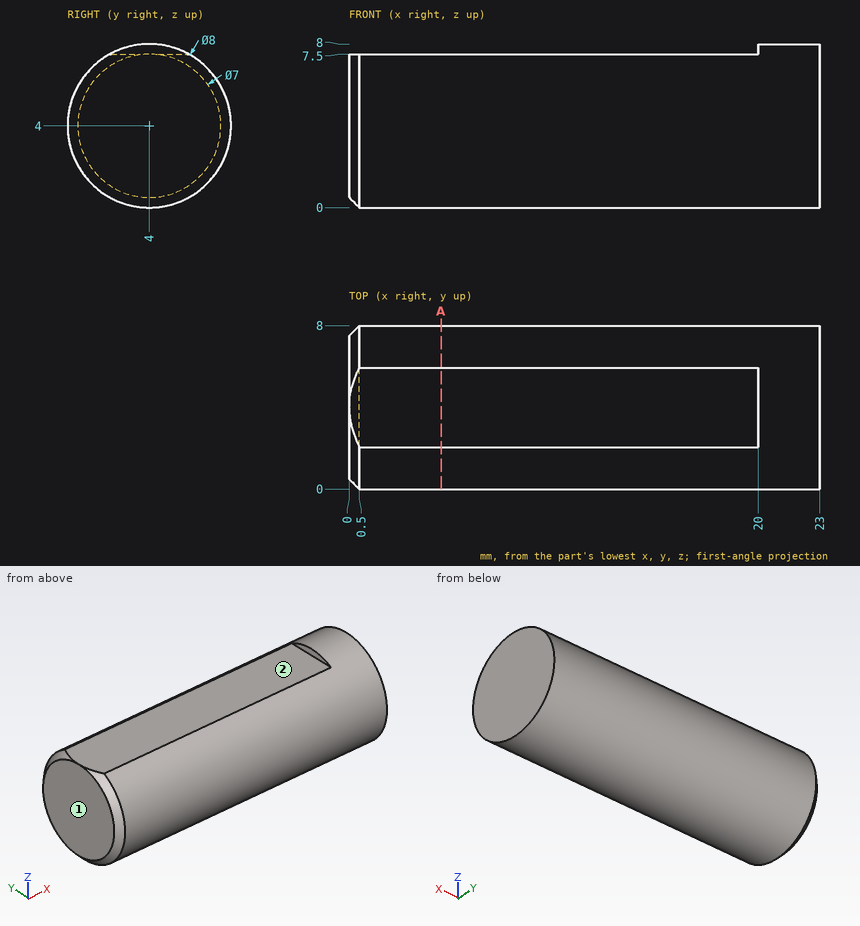
The drawing under review shows one solid part. Ordinate dimensions are in mm from its lowest x, y, z. A direction names the side the tool comes from. Coordinates: 2 decimals unless noted, no trailing zeros. Order: outer loops, then holes, each group sorted by start corner. A loop starts at its lowest first (then second) coordinate and runs counter-clockwise, first axis right, second up. Notation, with made-up numbers: (80, 43) -> (112, 43) arc R23 cw to (112, 69) -> close; hole circle Ø11 at (50.5, 8). An arc over 180 degrees is marked (long way). Answer in a Markdown table with one row per item. Add a question column.
Item 1: Clearance check with a flat-ended pin moving along its axis: pin 1 (1.9 mm diameter, centred on x = 9.5, y = 4, fed in from +Z). State where the tip first meets the part, or that it passes through.
Item 2: Machinability: for the marked faces 1 and 2, which of the approach directions +Z, -Z, +X, -X, +Y, -Y give a long, thin tool a straight path to every point of the face, cutting with its end or side? Answer none if there is none.
Item 3: To check wall thickness, follow probe 1 along Y at (x, z) = (11.5, 0.5) (1 decimal); probe 2 along X at (y, z) = (0.5, 3.25); probe 3 along Z at (x, y) = (3.5, 3). State the ranges of each line that lie inside material, in increasing order.
Item 4: We need section A-A on x = 4.5. Write out the cut boundary in (y, z).
Final values:
| question | item | result |
|---|---|---|
| 1 | pin 1 | stops at z = 7.5 |
| 2 | face 1 | +Z, -Z, -X, +Y, -Y |
| 2 | face 2 | +Z, -X, +Y, -Y |
| 3 | probe 1 | y = 2.1 to 5.9 |
| 3 | probe 2 | x = 0.08 to 23 |
| 3 | probe 3 | z = 0.13 to 7.5 |
| 4 | outline | (2.06, 7.5) arc R4 ccw (long way) to (5.94, 7.5) -> close |
